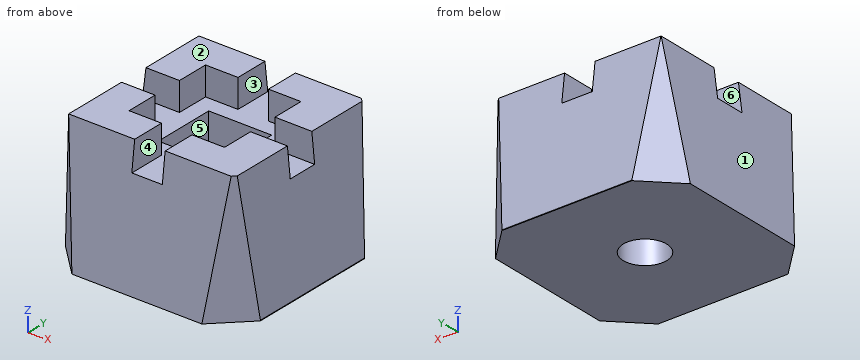
from build123d import *

# Parameters (mm, degrees)
F0_W      = 304.8
F0_H      = 304.8
F1_DEPTH  = 203.2
F2_W      = 149.225
F2_H      = 149.225
F3_DEPTH  = 44.45
F4_W      = 47.625
F4_H      = 77.7875
F4_W_2    = 77.7875
F4_H_2    = 47.625
F5_DEPTH  = 44.45
F6_SIZE   = 50.8
F7_R      = 33.9315428176
F8_DEPTH  = 158.751
F9_W      = 98.425
F9_H      = 98.425
F9_R      = 33.9315428176
F10_DEPTH = 76.2
F12_DEPTH = 304.801
F14_DEPTH = 304.801


with BuildPart() as f1:
    # F0 (on Top) → F1 (new body)
    with BuildSketch(Plane.XY):
        with Locations((152.4, 152.4)):
            Rectangle(F0_W, F0_H)
    extrude(amount=F1_DEPTH)

    # F2 (on face) → F3 (cut)
    with BuildSketch(Plane.XY.offset(203.2)):
        with Locations((152.4, 152.4)):
            Rectangle(F2_W, F2_H)
    extrude(amount=-F3_DEPTH, mode=Mode.SUBTRACT)

    # F4 (on face) → F5 (cut)
    with BuildSketch(Plane.XY.offset(203.2)):
        with Locations((152.4, 265.90625)):
            Rectangle(F4_W, F4_H)
        with Locations((152.4, 38.89375)):
            Rectangle(F4_W, F4_H)
        with Locations((265.90625, 152.4)):
            Rectangle(F4_W_2, F4_H_2)
        with Locations((38.89375, 152.4)):
            Rectangle(F4_W_2, F4_H_2)
    extrude(amount=-F5_DEPTH, mode=Mode.SUBTRACT)

    # F6
    f6_edges = [f1.edges().sort_by_distance(p)[0] for p in [
        (304.8, 0, 101.6),
        (304.8, 304.8, 101.6),
        (0, 0, 101.6),
        (0, 304.8, 101.6),
    ]]
    chamfer(f6_edges, length=F6_SIZE)

    # F7 (on face) → F8 (cut, through all)
    with BuildSketch(Plane.XY.offset(158.75)):
        with Locations((152.4, 152.4)):
            Circle(F7_R)
    extrude(amount=-F8_DEPTH, mode=Mode.SUBTRACT)

    # F9 (on face) → F10 (cut)
    with BuildSketch(Plane.XY.offset(158.75)):
        with Locations((152.4, 152.4)):
            Rectangle(F9_W, F9_H)
        with Locations((152.4, 152.4)):
            Circle(F9_R, mode=Mode.SUBTRACT)
    extrude(amount=-F10_DEPTH, mode=Mode.SUBTRACT)

    # F11 (on face) → F12 (cut, through all)
    with BuildSketch(Plane.XZ):
        Polygon((0, 203.2701924012), (0, 0), (25.4, 203.2701924012), align=None)
        Polygon((284.6523523331, 203.4087479115), (304.8951923847, 0), (304.8951923847, 203.4087479115), align=None)
    extrude(amount=-F12_DEPTH, mode=Mode.SUBTRACT)

    # F13 (on face) → F14 (cut, through all)
    with BuildSketch(Plane.YZ.offset(304.8)):
        Polygon((0, 203.302398324), (0, 0), (25.4, 203.302398324), align=None)
        Polygon((279.5212098122, 203.6561071873), (304.9212098122, 0), (304.9212098122, 203.6561071873), align=None)
    extrude(amount=-F14_DEPTH, mode=Mode.SUBTRACT)


solid = f1.part
Geometry check sheet. Reference: the model listing, model coordinates, mm. Face numbers are marked on the shaded views. A direction names the side the tool comes from. Coordinates: 2 decimals unless noted, no trailing zeros. Order: outer loops, then holes, each group sorted by start corner. A loop starts at its lowest first (then second) coordinate and runs counter-clockwise, first axis right, second up. Notation, with made-up numbers: (25, -4.75) - (36, -4.75) arc R18 ccw to (36, 12.25) - close; hole circle Ø4 at (79.25, 59). An arc over 180 degrees is marked (long way). One line per item, written item: value.
(1) Thickness scan on probe 1 along Z at (x, y) = (20, 163); probe 2 along X at (y, z) = (42, 178); probe 3 along X at (y, z) = (152, 56). Record the ranges inside material, lowest first. Write a range as from..to.
Data:
probe 1: z = 0..158.75
probe 2: x = 22.24..128.59, 176.21..287.18
probe 3: x = 7..118.47, 186.33..299.32
(2) Sectioned sample at D-D (x = 191). Enter the section's corners in (y, z).
Data:
outline: (0, 0) - (304.8, 0) - (304.8, 0.97) - (279.58, 203.2) - (227.01, 203.2) - (227.01, 158.75) - (201.61, 158.75) - (201.61, 82.55) - (103.19, 82.55) - (103.19, 158.75) - (77.79, 158.75) - (77.79, 203.2) - (25.39, 203.2) - close
(3) Access from +Z, -Z, +X, -X, +Y, -Y to the whole of each face (thin tool, end or side, straight path). Record for the marked faces 4, 5 and 6.
Data:
face 4: +Z, +Y, -Y
face 5: +Z
face 6: +Z, +X, -X
(4) Release check for a two-part mould opening along X. For the marked faces 1, 2 and 3 record: +X half, -X half, draft (parallel to the pull), parting line (faces both ways), or undercut.
Data:
face 1: -X half
face 2: draft
face 3: undercut
(5) Sectioned sample at C-C (z = 29). Enter the section's corners in (x, y), and give its area (3 significant figures).
Data:
outline: (3.62, 47.18) - (47.18, 3.62) - (257.62, 3.62) - (302.01, 48.01) - (302.01, 256.79) - (257.5, 301.3) - (47.3, 301.3) - (3.62, 257.62) - close; hole circle Ø67.86 at (152.4, 152.4)
area: 81,300 mm^2
(6) Depth check by flat-ended pin: pin 1 Ø6 at (x, z) = (61, 123.5) entering from +Y; pin 2 Ø13.5 at (x, z) = (52.5, 173) entering from -Y; pin 3 Ø13.5 at (x, z) = (209.5, 188) entering from -Y. Enter the tip coordinate at first touch or a pass-through.
Data:
pin 1: stops at y = 289.89
pin 2: stops at y = 20.77
pin 3: stops at y = 22.64
(7) Sectioned sample at B-B (y = 152.4). Enter the section's corners in (x, z).
Data:
outline: (0, 0) - (118.47, 0) - (118.47, 82.55) - (103.19, 82.55) - (103.19, 158.75) - (19.84, 158.75) - close; (186.33, 0) - (304.8, 0) - (304.8, 0.96) - (289.1, 158.75) - (201.61, 158.75) - (201.61, 82.55) - (186.33, 82.55) - close
(8) Sectioned sample at A-A (x = 152.4). Enter the section's corners in (y, z).
Data:
outline: (0, 0) - (118.47, 0) - (118.47, 82.55) - (103.19, 82.55) - (103.19, 158.75) - (19.83, 158.75) - close; (186.33, 0) - (304.8, 0) - (304.8, 0.97) - (285.12, 158.75) - (201.61, 158.75) - (201.61, 82.55) - (186.33, 82.55) - close
